Geometry check sheet. Reference: the model listing, model coordinates, mm. Face numbers are marked on the shaded views. A direction names the side the tool comes from. Give positions to 0.01 mm unless a question says otherwise; leave off trailing zeros. Write each loop counter-clockwise with the first axis right and the second up, starting at its lowest first coordinate (ties: lowest second). Pieces come first, ordered by that corner, then holes. Notation, with made-up numbers: (45.5, -38.5) -> (57.5, -38.5) arc R20 cw to (57.5, -4.5) -> close; hole circle Ø8 at (43.25, 10). An arc over 180 degrees is marked (long way). Use a Markdown table: item, result. Add a question column.
from build123d import *

# Parameters (mm, degrees)
SKETCH1_W           = 24
SKETCH1_H           = 12
SKETCH1_R           = 3.175
BOSS_EXTRUDE1_DEPTH = 3
SKETCH3_W           = 3
SKETCH3_H           = 12
BOSS_EXTRUDE2_DEPTH = 26
FILLET1_R           = 1
CHAMFER1_SIZE       = 0.3


# Read off the part's stored shape, not the designer's step: Mirror1
with BuildPart() as part:
    # Sketch1 → Boss-Extrude1 (new body)
    with BuildSketch(Plane.XY):
        Rectangle(SKETCH1_W, SKETCH1_H)
        Circle(SKETCH1_R, mode=Mode.SUBTRACT)
    extrude(amount=BOSS_EXTRUDE1_DEPTH)

    # Sketch3 → Boss-Extrude2 (add)
    with BuildSketch(Plane.XY):
        with Locations((-13.5, 0)):
            Rectangle(SKETCH3_W, SKETCH3_H)
    extrude(amount=BOSS_EXTRUDE2_DEPTH)

    # Fillet1
    fillet1_edges = [part.edges().sort_by_distance(p)[0] for p in [
        (-12, 0, 3),
        (0, -6, 3),
        (-15, 0, 0),
        (-15, 6, 13),
        (-15, -6, 13),
        (-12, -6, 14.5),
        (-12, 6, 14.5),
        (-15, 0, 26),
        (-13.5, -6, 26),
        (-12, 0, 26),
        (-13.5, 6, 26),
        (-1.5, -6, 0),
        (-1.5, 6, 0),
        (0, 6, 3),
    ]]
    fillet(fillet1_edges, radius=FILLET1_R)

    # Mirror1: part across plane


with BuildPart() as part_1:
    add(part.part)
    add(part.part.mirror(Plane(origin=(0, 0, 0), x_dir=(0, 0, 1), z_dir=(1, 0, 0))))

    # Chamfer1
    chamfer1_edges = [part_1.edges().sort_by_distance(p)[0] for p in [
        (-3.175, 0, 0),
        (-3.175, 0, 3),
    ]]
    chamfer(chamfer1_edges, length=CHAMFER1_SIZE)


solid = part_1.part
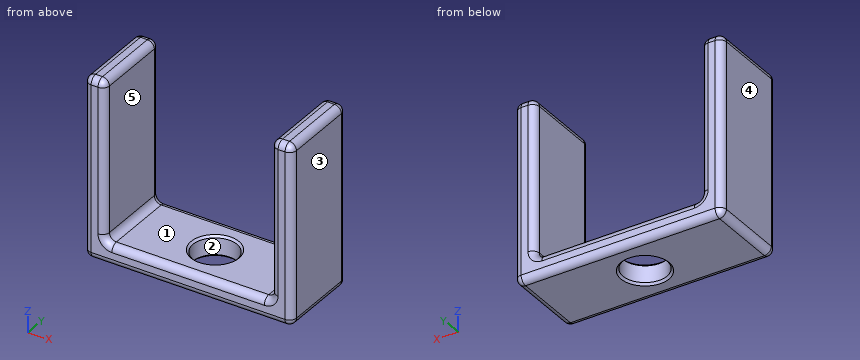
1) Draft check along X on the marked faces 3, 4 and 5. Enter one of: +X half, -X half, draft (parallel to the pull), parting line (faces both ways), or undercut.
2) Material ranges on probe 1 along X at (y, z) = (5, 23); probe 2 along Y at (x, z) = (0, 1.4) (3 decimals); probe 3 along Z at (x, y) = (11, 2.5), recorded low to high. Write a range as [from, to].
3) Sectioned sample at D-D, the plane x = -10.25. Enter the section's corners in (y, z), and give its area (3 significant figures).
4) Sectioned sample at A-A, the plane y = 0. Enter the section's corners in (x, z) (3 decimals).
5) Gauge pin test, flat end, axial feed: P1, Ø6, axis at x = 6, y = 2, coming from the +Z side. Record the tip position at first contact, or that the pin passes through.
6) Sectioned sample at B-B, the plane x = 0. Enter the section's corners in (y, z) (3 decimals), and give its area (3 significant figures).
7) Tool access check on the marked faces 1 and 2. Record the directions out of +Z, -Z, +X, -X, +Y, -Y that give a thin tool (end or side, any length) a straight path to the whole face; none if there is none.
8) Sectioned sample at C-C, the plane z = 4.75. Enter the section's corners in (x, y).
Check values:
| question | item | result |
|---|---|---|
| 1 | face 3 | +X half |
| 1 | face 4 | -X half |
| 1 | face 5 | undercut |
| 2 | probe 1 | [-15, -12], [12, 15] |
| 2 | probe 2 | [-6, -3.175], [3.175, 6] |
| 2 | probe 3 | [0, 3] |
| 3 | outline | (-6, 1) arc R1 ccw to (-5, 0) -> (5, 0) arc R1 ccw to (6, 1) -> (6, 2) arc R1 ccw to (5, 3) -> (-5, 3) arc R1 ccw to (-6, 2) -> close |
| 3 | area | 35.1 mm² |
| 4 | outline | (-15, 1) arc R1 ccw to (-14, 0) -> (-3.475, 0) -> (-3.175, 0.3) -> (-3.175, 2.7) -> (-3.475, 3) -> (-11, 3) arc R1 cw to (-12, 4) -> (-12, 25) arc R1 ccw to (-13, 26) -> (-14, 26) arc R1 ccw to (-15, 25) -> close; (3.175, 0.3) -> (3.475, 0) -> (14, 0) arc R1 ccw to (15, 1) -> (15, 25) arc R1 ccw to (14, 26) -> (13, 26) arc R1 ccw to (12, 25) -> (12, 4) arc R1 cw to (11, 3) -> (3.475, 3) -> (3.175, 2.7) -> close |
| 5 | P1 | z = 3 |
| 6 | outline | (-6, 1) arc R1 ccw to (-5, 0) -> (-3.475, 0) -> (-3.175, 0.3) -> (-3.175, 2.7) -> (-3.475, 3) -> (-5, 3) arc R1 ccw to (-6, 2) -> close; (3.175, 0.3) -> (3.475, 0) -> (5, 0) arc R1 ccw to (6, 1) -> (6, 2) arc R1 ccw to (5, 3) -> (3.475, 3) -> (3.175, 2.7) -> close |
| 6 | area | 15.9 mm² |
| 7 | face 1 | +Z, +Y, -Y |
| 7 | face 2 | +Z, -Z |
| 8 | outline | (-15, -5) arc R1 ccw to (-14, -6) -> (-13, -6) arc R1 ccw to (-12, -5) -> (-12, 5) arc R1 ccw to (-13, 6) -> (-14, 6) arc R1 ccw to (-15, 5) -> close; (12, -5) arc R1 ccw to (13, -6) -> (14, -6) arc R1 ccw to (15, -5) -> (15, 5) arc R1 ccw to (14, 6) -> (13, 6) arc R1 ccw to (12, 5) -> close |
